Read the model definition and answer for the solid it produces. Units are mm, in the model's axes. A direction names the side the tool comes from. Coordinates: 2 decimals unless noted, no trailing zeros. Order: outer loops, then holes, each group sorted by start corner. A loop starts at its lowest first (then second) coordinate and runs counter-clockwise, first axis right, second up. Notation, with made-up numbers: M 36,49.5 L 80,49.5 A34 ccw 80,80.5 Z; hole C -28,76 d10. An arc over 180 degrees is marked long. Use a Markdown table: item, result. Add a question column.
1) For faces 1 (the face through (4, 2, -6)), 2 (the face through (0, 2.7, -1.6)), determine the directions among +Z, -Z, +X, -X, +Y, -Y from which every point of the face is accessible in a straight line to the end or side of a thin tool.
2) Each of these flat-tipped pins is pushed along its axis until it touches: pin 1 Ø5 at (x, y) = (6, 5.5) entering from +Z; pin 2 Ø2.5 at (x, z) = (5, -5) entering from +Y; pin 3 Ø4 at (y, z) = (3, -0.5) entering from -X; pin 4 Ø2.5 at (x, y) = (3.5, 7) entering from -Z. Where does it stop, or does it pass through?
3) Find section A-A on x = 3. Write down the section's boundary in (y, z), plus the area to 3 significant figures.
4) Find section B-B on y = 7.75. Write down the section's boundary in (x, z).
5) Find the intervals of material crossed by probe 1 along Y at (x, z) = (1.75, -9.25); probe 2 along Y at (x, z) = (3, -0.5); probe 3 along Z at (x, y) = (4.75, 6), in increasing order. Write a range as [from, to].
Autodesk Inventor part; units mm, degrees
ref_plane "Work Plane2" through (10, 0, 0) normal (-0.5774, 0.5774, -0.5774) x (0.7071, 0, -0.7071)
ref_plane "YZ Plane" through (0, 0, 0) normal (1, 0, 0) x (0, 1, 0)
ref_plane "XZ Plane" through (0, 0, 0) normal (0, 1, 0) x (-1, 0, 0)
sketch "Sketch1" plane through (0, 0, 0) normal (1, 0, 0) x (0, 1, 0)
  line L0 (0, 0) -> (10, 0)
  line L1 (0, 0) -> (0, -10)
  line L2 (10, 0) -> (10, -10)
  line L3 (10, -10) -> (0, -10)
  dimension "d0" = 10
  dimension "d1" = 10
extrude "Extrusion1" add sketch "Sketch1" along normal blind 10
shell "Shell1" thickness 2 removed faces 3 at (3.3333, 10, -3.3333) at (3.3333, 6.6667, -10) at (0, 3.3333, -3.3333)
ref_plane "Work Plane2" through (10, 0, 0) normal (-0.5774, 0.5774, -0.5774) x (0.7071, 0, -0.7071)
ref_plane "Work Plane1" through (0, 10, -2) normal (-0.5774, 0.5774, -0.5774) x (0.7071, 0, -0.7071)
sketch "Sketch2" plane through (10, 0, 0) normal (-0.5774, 0.5774, -0.5774) x (0.7071, 0, -0.7071)
  line L0 (0, -8.165) -> (0, 0)
  line L1 (-7.0711, 4.0825) -> (0, 0)
  line L2 (0, 0) -> (7.0711, 4.0825)
  line L3 (0, -6.532) -> (0, 0)
  circle A0 centre (0, 0) radius 1.5
  dimension "d5" = 3
extrude "Extrusion2" add sketch "Sketch2" along normal up to next
sketch "Sketch3" plane through (10, 0, 0) normal (0.5774, -0.5774, 0.5774) x (0.7071, 0, -0.7071)
  point P0 (-7.0711, -4.0825)
sketch "Sketch4" plane through (10, 0, 0) normal (0.5774, -0.5774, 0.5774) x (0.7071, 0, -0.7071)
  circle A0 centre (0, 0) radius 1.5
  point P0 (-7.0711, -4.0825)
extrude "Extrusion3" add sketch "Sketch4" along normal blind 4
fillet "Fillet1" radius 0.5 1 edges at (11.2487, -2.3094, 3.3701)
properties part number "Corners"
Check result:
| question | item | result |
|---|---|---|
| 1 | face 1 | -Z, -X, +Y |
| 1 | face 2 | +Z, -Z, -X, +Y, -Y |
| 2 | pin 1 | stops at z = 0 |
| 2 | pin 2 | stops at y = 2 |
| 2 | pin 3 | stops at x = 0 |
| 2 | pin 4 | stops at z = -2 |
| 3 | outline | M 0,-10 L 2,-10 L 2,-2 L 10,-2 L 10,0 L 0,0 Z |
| 3 | area | 36.0 mm2 |
| 4 | outline | M 0,-2 L 8,-2 L 8,-10 L 10,-10 L 10,0 L 0,0 Z |
| 5 | probe 1 | y = [0, 2] |
| 5 | probe 2 | y = [0, 10] |
| 5 | probe 3 | z = [-2, 0] |
